Model file for the job. Use its own axes, mm. Round coordinates to 2 decimals unless told otherwise and drop trailing zeros. Write each loop counter-clockwise with the first axis right and the second up, starting at its lowest first coordinate (ties: lowest second). Pieces come first, ordered by that corner, then holes.
Autodesk Fusion 360 part; units mm, degrees
sketch "Sketch1" plane through (0, 0, 0) normal (0, 0, 1) x (1, 0, 0)
  line L0 (120.65, 120.65) -> (-120.65, 120.65)
  line L1 (-120.65, 120.65) -> (-120.65, -120.65)
  line L2 (-120.65, -120.65) -> (120.65, -120.65)
  line L3 (120.65, -120.65) -> (120.65, 120.65)
  line L4 (120.65, 120.65) -> (-120.65, -120.65) construction
  line L5 (-120.65, 120.65) -> (120.65, -120.65) construction
  dimension "d10" = 241.3
  dimension "d11" = 241.3
extrude "Extrude1" add sketch "Sketch1" along normal blind 2.54
sketch "Sketch2" plane through (0, 0, 2.54) normal (0, 0, 1) x (1, 0, 0)
  line L0 (120.65, -120.65) -> (120.65, 120.65)
  line L1 (120.65, 120.65) -> (-120.65, 120.65)
  line L2 (-120.65, 120.65) -> (-120.65, -120.65)
  line L3 (-120.65, -120.65) -> (120.65, -120.65)
  line L4 (110.49, 110.49) -> (-110.49, 110.49)
  line L5 (-110.49, 110.49) -> (-110.49, -110.49)
  line L6 (-110.49, -110.49) -> (110.49, -110.49)
  line L7 (110.49, -110.49) -> (110.49, 110.49)
  line L8 (110.49, 110.49) -> (-110.49, -110.49) construction
  line L9 (-110.49, 110.49) -> (110.49, -110.49) construction
  dimension "d14" = 220.98
  dimension "d15" = 220.98
sketch "Sketch3" plane through (0, 0, 2.54) normal (0, 0, 1) x (1, 0, 0)
  line L0 (110.49, 110.49) -> (-110.49, 110.49)
  line L1 (110.49, -110.49) -> (110.49, 110.49)
  line L2 (-110.49, -110.49) -> (110.49, -110.49)
  line L3 (-110.49, 110.49) -> (-110.49, -110.49)
  line L4 (-110.49, 110.49) -> (-85.09, 110.49)
  line L5 (-85.09, 110.49) -> (-85.09, 85.09)
  line L6 (-85.09, 85.09) -> (-110.49, 85.09)
  line L7 (-110.49, 85.09) -> (-110.49, 110.49)
  dimension "d16" = 25.4
  dimension "d17" = 25.4
sketch "Sketch4" plane through (0, 0, 2.54) normal (0, 0, 1) x (1, 0, 0)
  line L0 (110.49, 110.49) -> (-110.49, 110.49)
  line L1 (110.49, -110.49) -> (110.49, 110.49)
  line L2 (-110.49, -110.49) -> (110.49, -110.49)
  line L3 (-110.49, 110.49) -> (-110.49, -110.49)
  line L4 (-110.49, 110.49) -> (-85.09, 110.49)
  line L5 (-85.09, 110.49) -> (-85.09, 85.09)
  line L6 (-85.09, 85.09) -> (-110.49, 85.09)
  line L7 (-110.49, 85.09) -> (-110.49, 110.49)
  dimension "d20" = 25.4
  dimension "d21" = 25.4
extrude "Grid First Cut" cut sketch "Sketch4" against normal blind 5.08 contours L0 L3 L4 L5 L6 L7
pattern_linear "R-Pattern1" count 8 spacing 27.94 along (1, 0, 0) count 8 spacing 27.94 along (0, -1, 0) of "Grid First Cut"
extrude "Extrude2" cut sketch "Sketch3" against normal blind 5.08
equation "surfaceWidth = 9.5 in"
equation "surfaceDepth = 9.5 in"
equation "surfaceThickness = 0.1 in"
equation "borderWidth = 0.4 in"
equation "gridOpeningX = 1 in"
equation "gridOpeningY = 1 in"
equation "gridWebWidth = 0.1 in"
equation "payloadWidth = surfaceWidth - ( 2 * borderWidth )"
equation "payloadDepth = surfaceDepth - ( 2 * borderWidth )"
equation "d10 = surfaceWidth"
equation "d11 = surfaceDepth"
equation "d12 = surfaceThickness"
equation "d14 = payloadWidth"
equation "d15 = payloadDepth"
equation "d16 = gridOpeningX"
equation "d17 = gridOpeningY"
equation "d20 = gridOpeningY"
equation "d21 = gridOpeningX"
equation "gridPitchX = gridOpeningX + gridWebWidth"
equation "d29 = gridPitchX"
equation "d30 = gridPitchX"
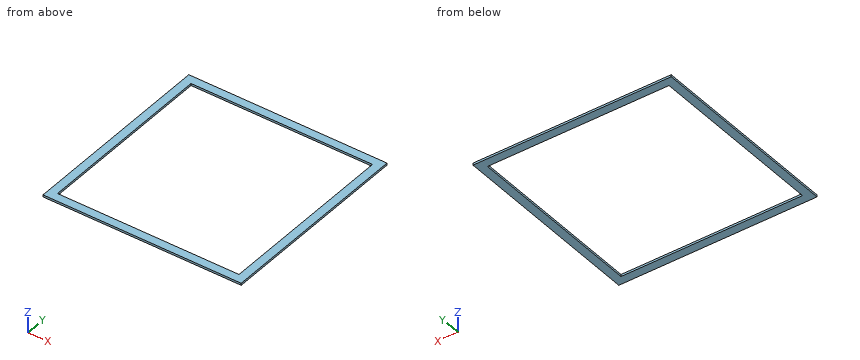
1) Cut at C-C on z = 0.75. List the corners of the cut face in (x, y).
2) Wall check: probe 1 along X at (y, z) = (12, 0.55). Give the ranges that are in metal, low to high.
3) Cut at A-A on y = -61. List the corners of the cut face in (x, z).
Result sheet:
1. outline: (-120.65, -120.65) - (120.65, -120.65) - (120.65, 120.65) - (-120.65, 120.65) - close; hole (-110.49, -110.49) - (110.49, -110.49) - (110.49, 110.49) - (-110.49, 110.49) - close
2. probe 1: x = -120.65 to -110.49, 110.49 to 120.65
3. outline: (-120.65, 0) - (-110.49, 0) - (-110.49, 2.54) - (-120.65, 2.54) - close; (110.49, 0) - (120.65, 0) - (120.65, 2.54) - (110.49, 2.54) - close
